Here's how the part is built. I have some questions about the finished solid (model axes, mm). Face numbers are marked on the shaded views. A direction names the side the tool comes from. Coordinates: 2 decimals unless noted, no trailing zeros. Write each loop counter-clockwise with the first axis right and the second up, starting at its lowest first coordinate (ties: lowest second). Pieces come first, ordered by that corner, then holes. Notation, with made-up numbers: (10.5, 74) -> (61.5, 74) arc R22 cw to (61.5, 113) -> close; hole circle Ø9 at (37.25, 63.5). An arc over 180 degrees is marked (long way). Use a Markdown table: item, result. Add a question column.
Item 1: Imagine slicing it at B-B, the plane x = -15.5. Write out the boundary of the cut face in (y, z).
Item 2: On a 3-axis mill with a long thin cutter (end or side, diameter ignored), from which of +Z, -Z, +X, -X, +Y, -Y can I reach the whole of each face in a straight line? I mean the marked faces 4, 5, 6, 7 and 8. Say none if no direction works.
Item 3: If I drill on line 1 along X through (y, z) = (-15.5, 18.2); line 2 along Y through (x, z) = (0, 16.4); line 3 along Z through (x, y) = (24, 21.5), over which ranges is the centre line in solid material (lowest first)? Write a range as from..to.
Item 4: Will these pins go through, and if not, where does the flat tip stop? pin 1 Ø6 at (x, z) = (9, 8) entering from +Y; pin 2 Ø10 at (x, y) = (25.5, 14.5) entering from -Z; pin 3 Ø4 at (y, z) = (-9, 5.5) entering from -X.
Item 5: Imagine slicing it at A-A, the plane y = 0. Write out the boundary of the cut face in (x, z).
Item 6: If we mould it in two halves opening along X, with no side actions, what happens to the marked faces 1, 2 and 3? For each: pulls with the +X half, pulls with the -X half, needs draft (parallel to the pull), parting line crosses it, or undercut.
Item 7: Imagine slicing it at C-C, the plane z = 10.5. Write out the boundary of the cut face in (x, y), and give its area (3 significant figures).
Item 8: Imagine slicing it at D-D, the plane x = 15.5. Count the separate pieces of the cut face and the enclosed holes in it, and give its area (3 significant figures).
```python
from build123d import *

# Parameters (mm, degrees)
CROQUIS1_R              = 1.7
SALIENTE_EXTRUIR1_DEPTH = 5
CROQUIS2_R              = 39.012383989
SALIENTE_EXTRUIR2_DEPTH = 20
CORTAR_EXTRUIR1_START   = -5
CROQUIS3_R              = 1.7
CROQUIS3_R_2            = 10
CORTAR_EXTRUIR1_DEPTH   = 5
CORTAR_EXTRUIR2_DEPTH   = 15
CHAFL_N1_SIZE           = 4.75
REDONDEO2_R             = 3.5
CROQUIS5_R              = 3.25
CORTAR_EXTRUIR3_DEPTH   = 15
MATRIZC1_COUNT          = 4
MATRIZC1_ANGLE          = 135
CROQUIS6_R              = 3.25
CORTAR_EXTRUIR4_DEPTH   = 2.5
CHAFL_N4_SIZE           = 2
CROQUIS8_R              = 1.75
CORTAR_EXTRUIR5_DEPTH   = 32.5


with BuildPart() as part:
    # Croquis1 → Saliente-Extruir1 (new body)
    with BuildSketch(Plane.XY):
        with BuildLine():
            Line((13.451293891, 42.926799862), (10.772509864, 36.459643134))
            ThreePointArc((10.772509864, 36.459643134), (38.017792496, 0), (10.772509864, -36.459643134))
            Line((10.772509864, -36.459643134), (13.451293891, -42.926799862))
            ThreePointArc((13.451293891, -42.926799862), (44.984969198, 0), (13.451293891, 42.926799862))
        make_face()
        with Locations((15.881362443, 38.341000599)):
            Circle(CROQUIS1_R, mode=Mode.SUBTRACT)
        with Locations((38.341000599, 15.881362443)):
            Circle(CROQUIS1_R, mode=Mode.SUBTRACT)
        with Locations((38.341000599, -15.881362443)):
            Circle(CROQUIS1_R, mode=Mode.SUBTRACT)
        with Locations((15.881362443, -38.341000599)):
            Circle(CROQUIS1_R, mode=Mode.SUBTRACT)
    extrude(amount=SALIENTE_EXTRUIR1_DEPTH)

    # Croquis2 → Saliente-Extruir2 (add)
    with BuildSketch(Plane(origin=(0, 0, 0), x_dir=(-1, 0, 0), z_dir=(0, 0, -1))):
        Circle(CROQUIS2_R)
    extrude(amount=-SALIENTE_EXTRUIR2_DEPTH)

    # Croquis3 → Cortar-Extruir1 (cut)
    with BuildSketch(Plane.XY.offset(20).offset(CORTAR_EXTRUIR1_START)):
        with Locations((-15.5, 15.5)):
            Circle(CROQUIS3_R)
        with Locations((15.5, 15.5)):
            Circle(CROQUIS3_R)
        with Locations((15.5, -15.5)):
            Circle(CROQUIS3_R)
        with Locations((-15.5, -15.5)):
            Circle(CROQUIS3_R)
        Circle(CROQUIS3_R_2)
        with BuildLine():
            Line((-20.5, 20), (-20.5, -20))
            Line((-20.5, -20), (3.526539614, -20))
            Line((3.526539614, -20), (6.774429386, -38.419698215))
            ThreePointArc((6.774429386, -38.419698215), (-39.012383989, 0), (6.774429386, 38.419698215))
            Line((6.774429386, 38.419698215), (3.526539614, 20))
            Line((3.526539614, 20), (-20.5, 20))
        make_face()
    extrude(amount=CORTAR_EXTRUIR1_DEPTH, mode=Mode.SUBTRACT)

    # Croquis4 → Cortar-Extruir2 (cut)
    with BuildSketch(Plane(origin=(0, 0, 0), x_dir=(-1, 0, 0), z_dir=(0, 0, -1))):
        with BuildLine():
            Line((-13.451293891, 42.926799862), (-11.155193297, 37.383522667))
            Line((-11.155193297, 37.383522667), (-9.803229729, 34.119593885))
            ThreePointArc((-9.803229729, 34.119593885), (-35.5, 0), (-9.803229729, -34.119593885))
            Line((-9.803229729, -34.119593885), (-11.155193297, -37.383522667))
            Line((-11.155193297, -37.383522667), (-13.451293891, -42.926799862))
            ThreePointArc((-13.451293891, -42.926799862), (44.984969198, 0), (-13.451293891, 42.926799862))
        make_face()
    extrude(amount=-CORTAR_EXTRUIR2_DEPTH, mode=Mode.SUBTRACT)

    # Chaflán1
    # the kernel refuses this chamfer: 4.75 mm, written as the material it takes off along each edge
    with BuildSketch(Plane(origin=(6.774429386, -38.419698215, 2.784505807), x_dir=(0.973158962162818, 0.2301339487389611, 0), z_dir=(0, 0, 1))) as chafl_n1_piece_1:
        with BuildLine():
            Line((4.498160378, 0), (CHAFL_N1_SIZE * 0.0576504165896, CHAFL_N1_SIZE * 0.998336831669))
            Line((CHAFL_N1_SIZE * 0.0576504165896, CHAFL_N1_SIZE * 0.998336831669), (0, 0))
            ThreePointArc((0, 0), (2.312261051, -0.064833001), (4.498160378, 0))
        make_face()
    extrude(amount=29.430988386, mode=Mode.SUBTRACT)
    with BuildSketch(Plane(origin=(6.774429386, 38.419698215, 2.784505807), x_dir=(0.9731589621628183, -0.23013394873896015, 0), z_dir=(0, 0, 1))) as chafl_n1_piece_2:
        with BuildLine():
            Line((4.498160378, 0), (CHAFL_N1_SIZE * 0.0576504165896, -CHAFL_N1_SIZE * 0.998336831669))
            Line((CHAFL_N1_SIZE * 0.0576504165896, -CHAFL_N1_SIZE * 0.998336831669), (0, 0))
            ThreePointArc((0, 0), (2.312261051, 0.064833001), (4.498160378, 0))
        make_face()
    extrude(amount=29.430988386, mode=Mode.SUBTRACT)

    # Redondeo2
    redondeo2_edges = [part.edges().sort_by_distance(p)[0] for p in [
        (5.949600542, 33.741861389, 17.5),
        (5.949600542, -33.741861389, 17.5),
        (3.526539614, 20, 17.5),
        (-20.5, 20, 17.5),
        (-20.5, -20, 17.5),
        (3.526539614, -20, 17.5),
        (13.451293891, -42.926799862, 2.5),
        (13.451293891, 42.926799862, 2.5),
    ]]
    fillet(redondeo2_edges, radius=REDONDEO2_R)

    # Croquis5 → Cortar-Extruir3 (cut)
    with BuildSketch(Plane.XY.offset(5)):
        with Locations((15.881362443, -38.341000599)):
            Circle(CROQUIS5_R)
    cortar_extruir3 = extrude(amount=CORTAR_EXTRUIR3_DEPTH, mode=Mode.SUBTRACT)

    # MatrizC1: Cortar-Extruir3 ×4 about axis
    matrizc1_axis = Axis((0, 0, 0), (0, 0, 1))
    for i in range(1, MATRIZC1_COUNT):
        add(cortar_extruir3.rotate(matrizc1_axis, i * MATRIZC1_ANGLE / (MATRIZC1_COUNT - 1)), mode=Mode.SUBTRACT)

    # Croquis6 → Cortar-Extruir4 (cut)
    with BuildSketch(Plane(origin=(0, 0, 15), x_dir=(-1, 0, 0), z_dir=(0, 0, -1))):
        with Locations((15.5, 15.5)):
            Circle(CROQUIS6_R)
        with Locations((15.5, -15.5)):
            Circle(CROQUIS6_R)
        with Locations((-15.5, -15.5)):
            Circle(CROQUIS6_R)
        with Locations((-15.5, 15.5)):
            Circle(CROQUIS6_R)
    extrude(amount=-CORTAR_EXTRUIR4_DEPTH, mode=Mode.SUBTRACT)

    # Chaflán4
    chafl_n4_edges = [part.edges().sort_by_distance(p)[0] for p in [
        (35.5, 0, 15),
    ]]
    chamfer(chafl_n4_edges, length=CHAFL_N4_SIZE)

    # Croquis8 → Cortar-Extruir5 (cut)
    with BuildSketch(Plane(origin=(0, 0, 0), x_dir=(-1, 0, 0), z_dir=(0, 0, -1))):
        with Locations((-40.5, 0)):
            Circle(CROQUIS8_R)
        with Locations(Location((-28.637824638, -28.637824638, 0), (0, 0, 13.876951429))):
            Circle(CROQUIS8_R)
        with Locations((-28.637824638, 28.637824638)):
            Circle(CROQUIS8_R)
    extrude(amount=-CORTAR_EXTRUIR5_DEPTH, mode=Mode.SUBTRACT)


solid = part.part
```
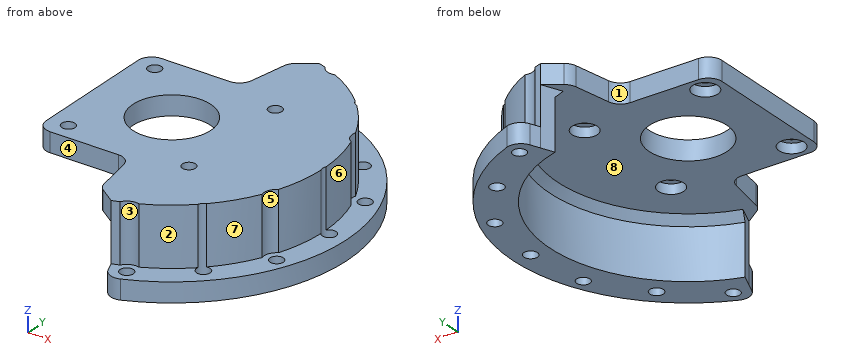
Ans:
| question | item | result |
|---|---|---|
| 1 | outline | (-20, 15) -> (-18.75, 15) -> (-18.75, 17.5) -> (-17.2, 17.5) -> (-17.2, 20) -> (-20, 20) -> close; (-13.8, 17.5) -> (-12.25, 17.5) -> (-12.25, 15) -> (12.25, 15) -> (12.25, 17.5) -> (13.8, 17.5) -> (13.8, 20) -> (-13.8, 20) -> close; (17.2, 17.5) -> (18.75, 17.5) -> (18.75, 15) -> (20, 15) -> (20, 20) -> (17.2, 20) -> close |
| 2 | face 4 | +Z, -Z, -X, -Y |
| 2 | face 5 | +Z, +X |
| 2 | face 6 | +Z, +X, +Y |
| 2 | face 7 | +Z, +X, -Y |
| 2 | face 8 | -Z, -X |
| 3 | line 1 | x = -20.5..-17.2, -13.8..13.8, 17.2..35.11 |
| 3 | line 2 | y = -20..-10, 10..20 |
| 3 | line 3 | z = 15..20 |
| 4 | pin 1 | stops at y = 37.38 |
| 4 | pin 2 | stops at z = 14.17 |
| 4 | pin 3 | stops at x = 33.75 |
| 5 | outline | (-20.5, 15) -> (-10, 15) -> (-10, 20) -> (-20.5, 20) -> close; (10, 15) -> (33.5, 15) -> (35.5, 13) -> (35.5, 0) -> (38.75, 0) -> (38.75, 20) -> (10, 20) -> close; (42.25, 0) -> (44.98, 0) -> (44.98, 5) -> (42.25, 5) -> close |
| 6 | face 1 | pulls with the -X half |
| 6 | face 2 | pulls with the +X half |
| 6 | face 3 | undercut |
| 7 | outline | (9.8, -34.12) -> (11.16, -37.38) arc R39.01 ccw to (13.04, -36.77) arc R3.25 cw to (16.78, -35.22) arc R39.01 ccw to (26.94, -28.22) arc R1.75 cw to (28.22, -26.94) arc R39.01 ccw to (35.22, -16.78) arc R3.25 cw to (36.77, -13.04) arc R39.01 ccw to (39, -0.9) arc R1.75 cw to (39, 0.9) arc R39.01 ccw to (36.77, 13.04) arc R3.25 cw to (35.22, 16.78) arc R39.01 ccw to (28.22, 26.94) arc R1.75 cw to (26.94, 28.22) arc R39.01 ccw to (16.78, 35.22) arc R3.25 cw to (13.04, 36.77) arc R39.01 ccw to (11.16, 37.38) -> (9.8, 34.12) arc R35.5 cw to start |
| 7 | area | 327 mm^2 |
| 8 | separate pieces | 5 |
| 8 | enclosed holes | 0 |
| 8 | area | 437 mm^2 |
